```python
from build123d import *

# Parameters (mm, degrees)
SKETCH_1_W      = 195.5
SKETCH_1_H      = 88
SKETCH_1_R      = 1.5
EXTRUDE_1_DEPTH = 10


with BuildPart() as part:
    # Эскиз1 → Бобышка-Вытянуть1 (new body)
    with BuildSketch(Plane(origin=(0, 0, 0), x_dir=(1, 0, 0), z_dir=(0, 1, 0))):
        with Locations((-50.25, 2.5)):
            Rectangle(SKETCH_1_W, SKETCH_1_H)
        with Locations(Location((-5.5, 15.5, 0), (0, 0, 270))):
            Circle(SKETCH_1_R, mode=Mode.SUBTRACT)
        with Locations(Location((5.5, 15.5, 0), (0, 0, 270))):
            Circle(SKETCH_1_R, mode=Mode.SUBTRACT)
        with Locations(Location((-5.5, -15.5, 0), (0, 0, 270))):
            Circle(SKETCH_1_R, mode=Mode.SUBTRACT)
        with Locations(Location((5.5, -15.5, 0), (0, 0, 270))):
            Circle(SKETCH_1_R, mode=Mode.SUBTRACT)
        with Locations(Location((-73, 36.5, 0), (0, 0, 270))):
            Circle(SKETCH_1_R, mode=Mode.SUBTRACT)
        with Locations(Location((-73, -36.5, 0), (0, 0, 270))):
            Circle(SKETCH_1_R, mode=Mode.SUBTRACT)
        with Locations(Location((-144.5, 40, 0), (0, 0, 270))):
            Circle(SKETCH_1_R, mode=Mode.SUBTRACT)
        Polygon((-13.5, 13), (-28, 12), (-48, 12), (-48, 13), (-68, 13), (-68, 31.5), (-78, 31.5), (-78, 22), (-128, 22), (-128, -22), (-78, -22), (-78, -31.5), (-68, -31.5), (-68, -13), (-48, -13), (-48, -12), (-28, -12), (-13.5, -13), (9.5, -13), (9.5, -20), (37.5, -20), (37.5, 20), (9.5, 20), (9.5, 13), align=None, mode=Mode.SUBTRACT)
    extrude(amount=EXTRUDE_1_DEPTH)


solid = part.part
```
Read the model definition and answer for the solid it produces. Units are mm, in the model's axes. A direction names the side the tool comes from. Coordinates: 2 decimals unless noted, no trailing zeros. Order: outer loops, then holes, each group sorted by start corner. A loop starts at its lowest first (then second) coordinate and runs counter-clockwise, first axis right, second up. Notation, with made-up numbers: (-24.75, 52.25) - (8.25, 52.25) arc R30 cw to (8.25, 88.25) - close; hole circle Ø4 at (43, 75.5). An arc over 180 degrees is marked (long way). Answer as a JSON object with one key per item and string values. Group by question number.
Item 1: Consider probe 1 along X at (y, z) = (3.25, 15.5); probe 2 along Z at (x, y) = (-73, 3.25); probe 3 along Z at (x, y) = (-29.5, 5.5). Determine where each line is inside the solid, lowest interval first. Write a range as from..to.
Item 2: Section A-A (x = -38) is taken. Give the vertices of the cut face in (y, z).
Item 3: Section B-B (z = -1) is taken. Give the vertices of the cut face in (x, y).
Item 4: A tool of negligible diameter and unlimited length cuts with its end or side. For faces 1 (the face through (-78, 5, -27)), 2 (the face through (-52, 0, -23)), from which of +Z, -Z, +X, -X, +Y, -Y can it reach the whole face along a straight path? Write none if from no direction.
Item 5: The mould has two halves that part along Z. Classify faces 3 (the face through (24, 5, -20)), 4 (the face through (-52, 5, -46.5)), 5 (the face through (-52, 5, 41.5)): +Z half, -Z half, draft (parallel to the pull), parting line (faces both ways), or undercut.
Item 6: A flat-ended cylindrical pin translates along its axis: P1, Ø4, axis at x = -53, z = 9.5, coming from the +Y side. Find the tip coordinate at first contact, or state that the pin passes through.
Item 7: Section C-C (y = 7.25) is taken. State how many separate pieces and enclosed holes the cut face has, plus the area to 3 significant figures.
Results are:
{
 "1": {"probe 1": "x = -148..-128, -68..-7, -4..4, 7..9.5, 37.5..47.5", "probe 2": "z = -46.5..-38, -35..-31.5, 31.5..35, 38..41.5", "probe 3": "z = -46.5..-12, 12..41.5"},
 "2": {"outline": "(0, -46.5) - (10, -46.5) - (10, -12) - (0, -12) - close; (0, 12) - (10, 12) - (10, 41.5) - (0, 41.5) - close"},
 "3": {"outline": "(-148, 0) - (-128, 0) - (-128, 10) - (-148, 10) - close; (37.5, 0) - (47.5, 0) - (47.5, 10) - (37.5, 10) - close"},
 "4": {"face 1": "+Y, -Y", "face 2": "+Z, -Z, +X, -X, -Y"},
 "5": {"face 3": "undercut", "face 4": "-Z half", "face 5": "+Z half"},
 "6": {"P1": "passes through"},
 "7": {"separate pieces": "1", "enclosed holes": "8", "area": "11,200 mm^2"}
}
